Geometry: final body of the model. Coordinates: model frame, mm. Round coordinates to 2 decimals unless told otherwise and drop trailing zeros. Loops run counter-clockwise (first coordinate to the right, second up) from the corner with the lowest first, then second, coordinate; pieces in that order, holes last. Notation, with made-up numbers: (-35.75, -14.5) - (21.25, -14.5) arc R19 cw to (21.25, 21.5) - close; hole circle Ø3 at (42, -1.75). An arc over 180 degrees is marked (long way). Answer as a JSON object with one key per item and string values. Group by question number.
Item 1: Section A-A (x = 78). Return the cut outline in (y, z), plus the area to 3 significant figures.
Item 2: First-contact query: pin 1 (1 mm diameter, centred on x = 111, y = -1.5, fed in from +Z); pin 2 (1.5 mm diameter, centred on x = 19.5, z = -1.5, fed in from -Y). Flat tips, straight axial feed; report the tip coordinate or a pass-through.
Item 3: Line query: line 1 (Y direction, x = 14, z = -0.1); line 2 (Z direction, x = 166, y = -0.3); line 3 (X direction, y = 0, z = -0.75). Output: solid intervals per line, ascending.
```python
from build123d import *

# Parameters (mm, degrees)
SKETCH1_R               = 2.25
BOSS_EXTRUDE1_DEPTH     = 180
FILLET1_R               = 0.75
CUT_EXTRUDE1_DEPTH      = 181.028122803
CUT_EXTRUDE1_DEPTH_BACK = 181.028122803
CAVITY1_OUTLINE_W       = 1
CAVITY1_OUTLINE_H       = 4.503251691


# Read off the part's stored shape, not the designer's step: Cavity1
with BuildPart() as part:
    # Sketch1 → Boss-Extrude1 (new body)
    with BuildSketch(Plane(origin=(0, 0, 0), x_dir=(0, 0, -1), z_dir=(1, 0, 0))):
        with Locations(Location((0, 0, 0), (0, 0, 180))):
            Circle(SKETCH1_R)
    extrude(amount=BOSS_EXTRUDE1_DEPTH)

    # Fillet1
    fillet1_edges = [part.edges().sort_by_distance(p)[0] for p in [
        (0, 0, -2.25),
    ]]
    fillet(fillet1_edges, radius=FILLET1_R)

    # Sketch2 → Cut-Extrude1 (cut, two sides: drawn at the far end of the back side and taken through both)
    with BuildSketch(Plane.XY.offset(-CUT_EXTRUDE1_DEPTH_BACK)):
        with BuildLine():
            Line((180, 2.25), (177.75, 2.25))
            ThreePointArc((177.75, 2.25), (179.340990258, 1.590990258), (180, 0))
            Line((180, 0), (180, 2.25))
        make_face()
        with BuildLine():
            Line((180, -2.25), (180, 0))
            ThreePointArc((180, 0), (179.340990258, -1.590990258), (177.75, -2.25))
            Line((177.75, -2.25), (180, -2.25))
        make_face()
    extrude(amount=CUT_EXTRUDE1_DEPTH + CUT_EXTRUDE1_DEPTH_BACK, mode=Mode.SUBTRACT)

    # Cavity1 outline → Cavity1 (revolve, cut)
    with BuildSketch(Plane(origin=(177.75, -0.001139824, -0.214423248), x_dir=(1, 0, 0), z_dir=(0, 0.005315692237830849, 0.9999858716082107))):
        with Locations((0.5, 0.001514697)):
            Rectangle(CAVITY1_OUTLINE_W, CAVITY1_OUTLINE_H)
    revolve(axis=Axis((177.75, -0.001139824, -0.214423248), (0, 0.9999858716082107, -0.005315692237830849)), mode=Mode.SUBTRACT)


solid = part.part
```
Values:
{
 "1": {"outline": "circle Ø4.5 at (0, 0)", "area": "15.9 mm^2"},
 "2": {"pin 1": "stops at z = 2.02", "pin 2": "stops at y = -2.12"},
 "3": {"line 1": "y = -2.25 to 2.25", "line 2": "z = -2.23 to 2.23", "line 3": "x = 0 to 176.91, 178.59 to 180"}
}
